from build123d import *

# Parameters (mm, degrees)
SKETCH1_W           = 63.5
SKETCH1_H           = 44.36533333
BOSS_EXTRUDE1_DEPTH = 1.5
SKETCH2_R           = 1.5
SKETCH2_W           = 14.1
SKETCH2_H           = 14.1
CUT_EXTRUDE1_DEPTH  = 78.477627748
SKETCH4_R           = 2.75
CUT_EXTRUDE2_DEPTH  = 1
FILLET1_R           = 2


with BuildPart() as part:
    # Sketch1 → Boss-Extrude1 (new body)
    with BuildSketch(Plane(origin=(0, 0, 0), x_dir=(1, 0, 0), z_dir=(0, 1, 0))):
        with Locations((31.75, 22.182666665)):
            Rectangle(SKETCH1_W, SKETCH1_H)
    extrude(amount=BOSS_EXTRUDE1_DEPTH)

    # Sketch2 → Cut-Extrude1 (cut, through all)
    with BuildSketch(Plane(origin=(0, 1.5, 0), x_dir=(1, 0, 0), z_dir=(0, 1, 0))):
        with Locations(Location((3.2, 41.16533333, 0), (0, 0, 270))):
            Circle(SKETCH2_R)
        with Locations(Location((60.3, 41.16533333, 0), (0, 0, 270))):
            Circle(SKETCH2_R)
        with Locations(Location((60.3, 3.2, 0), (0, 0, 270))):
            Circle(SKETCH2_R)
        with Locations(Location((3.2, 3.2, 0), (0, 0, 270))):
            Circle(SKETCH2_R)
        with Locations((12.7, 31.70766667)):
            Rectangle(SKETCH2_W, SKETCH2_H)
        with Locations((31.75, 31.70766667)):
            Rectangle(SKETCH2_W, SKETCH2_H)
        with Locations((50.8, 31.70766667)):
            Rectangle(SKETCH2_W, SKETCH2_H)
        with Locations((12.7, 12.65766667)):
            Rectangle(SKETCH2_W, SKETCH2_H)
        with Locations((31.75, 12.65766667)):
            Rectangle(SKETCH2_W, SKETCH2_H)
        with Locations((50.8, 12.65766667)):
            Rectangle(SKETCH2_W, SKETCH2_H)
    extrude(amount=-CUT_EXTRUDE1_DEPTH, mode=Mode.SUBTRACT)

    # Sketch4 → Cut-Extrude2 (cut)
    with BuildSketch(Plane(origin=(0, 1.5, 0), x_dir=(1, 0, 0), z_dir=(0, 1, 0))):
        with Locations(Location((3.2, 41.16533333, 0), (0, 0, 270))):
            Circle(SKETCH4_R)
        with Locations(Location((60.3, 41.16533333, 0), (0, 0, 270))):
            Circle(SKETCH4_R)
        with Locations(Location((60.3, 3.2, 0), (0, 0, 270))):
            Circle(SKETCH4_R)
        with Locations(Location((3.2, 3.2, 0), (0, 0, 270))):
            Circle(SKETCH4_R)
    extrude(amount=-CUT_EXTRUDE2_DEPTH, mode=Mode.SUBTRACT)

    # Fillet1
    fillet1_edges = [part.edges().sort_by_distance(p)[0] for p in [
        (0, 0.75, -44.36533333),
        (63.5, 0.75, -44.36533333),
        (63.5, 0.75, 0),
        (0, 0.75, 0),
    ]]
    fillet(fillet1_edges, radius=FILLET1_R)


solid = part.part
Here's how the part is built. I have some questions about the finished solid (model axes, mm). A direction names the side the tool comes from. Round coordinates to 2 decimals unless told otherwise and drop trailing zeros. Write each loop counter-clockwise with the first axis right and the second up, starting at its lowest first coordinate (ties: lowest second). Pieces come first, ordered by that corner, then holes.
1. Suppose I cut it at D-D (y = 1.05). State how many separate pieces and enclosed holes the cut face has, and give its area (3 significant figures).
2. I need wall thicknesses on L1, parallel to Z at x = 25.5, y = 0.5; L2, parallel to X at y = 0.7, z = -3.2; L3, parallel to X at y = 0.45, z = -38.5. Which ranges of each line are inside material? Lowest first, please.
3. If we mould it in two halves opening along X, with no side actions, what happens to faces 4 (the cylindrical face through (62.899, 0.76, -43.795)), 5 (the flat face through (19.75, 1, -32)), 6 (the flat face through (31, 1, -44.365))? For each: released by +X, released by -X, zero draft, split by the parting line, or undercut.
4. Suppose I cut it at C-C (z = -3.2). List the corners of the cut face in (x, y) for me, and give its area (4 significant figures).
5. Suppose I cut it at A-A (x = 60.3). List the corners of the cut face in (y, z) for me.
6. Suppose I cut it at B-B (z = -27). List the corners of the cut face in (x, y) for me, and give its area (3 significant figures).
7. For faces 1 (the flat face through (59, 0.5, -2)), 2 (the flat face through (43.75, 1, -13)), 3 (the cylindrical face through (0.57, 0.76, -0.6)), which set-ups out of +Z, -Z, +X, -X, +Y, -Y let a thin tool reach every point of the face, with its end or its side?
Answer sheet:
1. separate pieces: 1
1. enclosed holes: 10
1. area: 1,530 mm2
2. L1: z = -44.37 to -38.76, -24.66 to -19.71, -5.61 to 0
2. L2: x = 0 to 0.45, 5.95 to 57.55, 63.05 to 63.5
2. L3: x = 0 to 5.65, 19.75 to 24.7, 38.8 to 43.75, 57.85 to 63.5
3. face 4: released by +X
3. face 5: undercut
3. face 6: zero draft
4. outline: (0, 0) - (1.7, 0) - (1.7, 0.5) - (0.45, 0.5) - (0.45, 1.5) - (0, 1.5) - close; (4.7, 0) - (58.8, 0) - (58.8, 0.5) - (57.55, 0.5) - (57.55, 1.5) - (5.95, 1.5) - (5.95, 0.5) - (4.7, 0.5) - close; (61.8, 0) - (63.5, 0) - (63.5, 1.5) - (63.05, 1.5) - (63.05, 0.5) - (61.8, 0.5) - close
4. area: 81.25 mm2
5. outline: (0, -44.37) - (1.5, -44.37) - (1.5, -43.92) - (0.5, -43.92) - (0.5, -42.67) - (0, -42.67) - close; (0, -39.67) - (0.5, -39.67) - (0.5, -38.42) - (1.5, -38.42) - (1.5, -5.95) - (0.5, -5.95) - (0.5, -4.7) - (0, -4.7) - close; (0, -1.7) - (0.5, -1.7) - (0.5, -0.45) - (1.5, -0.45) - (1.5, 0) - (0, 0) - close
6. outline: (0, 0) - (5.65, 0) - (5.65, 1.5) - (0, 1.5) - close; (19.75, 0) - (24.7, 0) - (24.7, 1.5) - (19.75, 1.5) - close; (38.8, 0) - (43.75, 0) - (43.75, 1.5) - (38.8, 1.5) - close; (57.85, 0) - (63.5, 0) - (63.5, 1.5) - (57.85, 1.5) - close
6. area: 31.8 mm2
7. face 1: +Y
7. face 2: +Y, -Y
7. face 3: +Z, -X, +Y, -Y
